Autodesk Inventor part; units mm, degrees
ref_plane "Work Plane2" through (8, 0, 0) normal (0, 0, 1) x (1, 0, 0)
ref_plane "Work Plane4" through (8, 0, 0) normal (0, 0, 1) x (1, 0, 0)
ref_plane "Work Plane5" through (11, -5, -9) normal (1, 0, 0) x (0, 1, 0)
ref_plane "Work Plane1" through (11, 2.9624, 8) normal (0, 0, -1) x (-1, 0, 0)
sketch "Sketch1" plane through (11, 2.9624, 8) normal (0, 0, -1) x (-1, 0, 0)
  arc A0 (0.0647, 1) -> (3.5, -0.2722) centre (5.5324, 10.4896) ccw
  line L0 (0, -2.9624) -> (0, 1)
  line L1 (3.5, -0.2722) -> (3.5, -2.9624)
  line L2 (0, -2.9624) -> (3.5, -2.9624)
  arc A1 (0, 1.0376) -> (11, 1) centre (5.5324, 10.4896) ccw
  line L3 (0, -7.9624) -> (0, 1.0376)
  line L4 (3.5, -0.2722) -> (3.5, -2.9624)
  line L5 (0, -2.9624) -> (3.5, -2.9624)
  line L6 (0, -2.9624) -> (0, 1.0376)
  arc A2 (0, 1.0376) -> (11, 1) centre (5.5324, 10.4896) ccw
  point P0 (11, -2.9624)
ref_plane "Work Plane2" through (8, 0, 0) normal (0, 0, 1) x (1, 0, 0)
ref_plane "Work Plane4" through (8, 0, 0) normal (0, 0, 1) x (1, 0, 0)
extrude "Extrusion1" add sketch "Sketch1" along normal up to surface (8 mm away)
ref_plane "Work Plane3" through (8, -5, 14.5) normal (-1, 0, 0) x (0, 0, 1)
ref_plane "Work Plane5" through (11, -5, -9) normal (1, 0, 0) x (0, 1, 0)
sketch "Sketch2" plane through (8, -5, 14.5) normal (-1, 0, 0) x (0, 0, 1)
  line L0 (-6.5, 5) -> (-14.5, 5)
  line L1 (-12, 5) -> (-12, 0)
  line L2 (-12, 5) -> (-12, 0)
  line L3 (-12, 5) -> (-9.4556, 5)
  line L4 (-12, 0) -> (-22.5, 0)
  line L5 (-22.5, 0) -> (-22.5, -26)
  line L6 (1.0444, 0) -> (1.0444, -26)
  line L7 (1.0444, -26) -> (-22.5, -26)
  line L8 (-22.5, 0) -> (-19.5, 0)
  line L9 (-19.5, 0) -> (-19.5, -3)
  line L10 (1.0444, -26) -> (1.0444, -23)
  line L11 (1.0444, -23) -> (-1.9556, -23)
  line L12 (-19.5, -3) -> (-1.9556, -3)
  line L13 (-1.9556, -3) -> (-1.9556, -23)
  line L14 (-1.9556, -23) -> (-19.5, -23)
  line L15 (-19.5, -23) -> (-19.5, -3)
  line L16 (1.0444, -26) -> (-0.9556, -26)
  line L17 (-0.9556, -26) -> (-2.9556, -26)
  line L18 (-22.5, 0) -> (-22.5, -4)
  line L19 (-22.5, -4) -> (-22.5, -2)
  line L20 (-22.5, -2) -> (-24.5, -2)
  line L21 (1.0444, 0) -> (1.0444, -4)
  line L22 (1.0444, -2) -> (3.0444, -2)
  arc A0 (-22.5, 0) -> (-22.5, -4) centre (-22.5, -2) ccw
  arc A1 (1.0444, -4) -> (1.0444, 0) centre (1.0444, -2) ccw
  line L23 (-9, 0) -> (-9, 5)
  line L24 (-12, 5) -> (-9, 5)
  line L25 (-9, 5) -> (-9, 0)
  line L26 (1.0444, 0) -> (-9, 0)
  line L27 (-22.5, -26) -> (-22.5, -24)
  line L28 (-22.5, -24) -> (-24.5, -24)
  line L29 (1.0444, -26) -> (1.0444, -24)
  line L30 (1.0444, -24) -> (3.0444, -24)
  line L31 (-22.5, -24) -> (-22.5, -22)
  line L32 (1.0444, -24) -> (1.0444, -22)
  arc A2 (-22.5, -22) -> (-22.5, -26) centre (-22.5, -24) ccw
  arc A3 (1.0444, -26) -> (1.0444, -22) centre (1.0444, -24) ccw
  line L33 (-19.5, -23) -> (-1.9556, -23)
  line L34 (-1.9556, -3) -> (-1.9556, -23)
  point P0 (-18.5, -26)
  dimension "d3" = 10.5
  dimension "d4" = 26
  dimension "d5" = 3
  dimension "d6" = 3
  dimension "d8" = 3
  dimension "d16" = 4
  dimension "d17" = 2
  dimension "d18" = 4
  dimension "d19" = 2
  dimension "d28" = 2
  dimension "d29" = 2
  dimension "d30" = 2
  dimension "d31" = 2
  dimension "d32" = 2
extrude "Extrusion2" add sketch "Sketch2" along normal up to surface (3.5 mm away) from surface at -3 contours L23 L26 L6 L11 L13 L12 L9 L4 L1 L0 | A1 L22 L6 | L22 A1 L6 | L9 L15 L14 L11 L6 L7 L5 L4 | L5 L20 A0 | A3 L30 L6 | L5 A0 L20 | A3 L6 L30 | L5 L28 A2 | L5 A2 L28
sketch "Sketch3" plane through (11, 0, 8) normal (1, 0, 0) x (0, 0, -1)
  arc A0 (-7.5444, -5) -> (-7.5444, -9) centre (-7.5444, -7) ccw
  arc A1 (16, -9) -> (16, -5) centre (16, -7) ccw
  circle A2 centre (16, -7) radius 1
  circle A3 centre (-7.5444, -7) radius 1
  arc A4 (-7.5444, -27) -> (-7.5444, -31) centre (-7.5444, -29) ccw
  arc A5 (16, -31) -> (16, -27) centre (16, -29) ccw
  circle A6 centre (16, -29) radius 1
  circle A7 centre (-7.5444, -29) radius 1
  point P0 (-5.5444, -31)
  dimension "d23" = 2
  dimension "d25" = 2
  dimension "d33" = 2
  dimension "d34" = 2
extrude "Extrusion3" cut sketch "Sketch3" against normal up to surface (3.5 mm away)
properties part number "back_pack_side_clip_in"
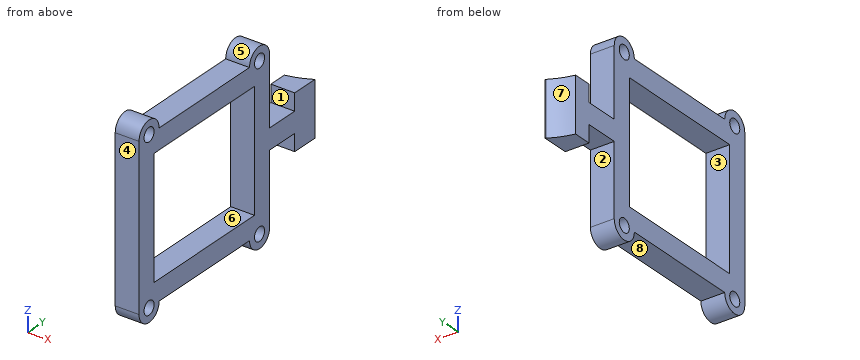
Input: part model. Units: mm. Frame: model coordinates. Face numbers are marked on the shaded views. A direction names the side the tool comes from. Give positions to 0.01 mm unless a question says otherwise; leave off trailing zeros. Write each loop counter-clockwise with the first axis right and the second up, starting at its lowest first coordinate (ties: lowest second). Pieces come first, ordered by that corner, then holes. Notation, with made-up numbers: (74.5, 11.5) - (103.5, 11.5) arc R21 cw to (103.5, 37.5) - close; hole circle Ø5 at (-20, 33). An arc over 180 degrees is marked (long way). Write item = value, one per line. Start each with the question number.
1. Section query A-A, the plane y = -29. Output: boundary loops of the cut face in (x, z), then the cut area to 3 significant figures.
2. Section query C-C, the plane x = 9.6. Output: boundary loops of the cut face in (y, z).
3. Section query B-B, the plane y = -23.5. Output: boundary loops of the cut face in (x, z), then the cut area to 3 significant figures.
4. First-contact query: pin 1 Ø1.8 at (x, z) = (10, 3.5) entering from +Y; pin 2 Ø1 at (x, z) = (10, -3.5) entering from +Y; pin 3 Ø2 at (x, y) = (10.5, -16) entering from +Z. Flat tips, straight axial feed; report the tip coordinate or a pass-through.
5. Section query D-D, the plane z = -5.5. Output: boundary loops of the cut face in (x, y), then the cut area to 3 significant figures.
6. Mould query, pull axis Z, two halves, no side actions, for the marked faces 5, 6, 7 and 8. Classes: released by +Z, released by -Z, zero draft, split by the parting line, or undercut.
7. Ray query, L1, parallel to Z at x = 7.95, y = -18.5; L2, parallel to Y at x = 8.45, z = 0.25; L3, parallel to Y at x = 10.75, z = 14.75. Return the intervals inside material, ascending.
8. Access query for the marked faces 1, 2, 3 and 4. Directions: +Z, -Z, +X, -X, +Y, -Y. A direction counts if a zero-diameter tool reaches every point of the face in a straight line with its end or side. Return the directions, or none.
Check sheet entries:
q1.outline = (7.5, -10) - (11, -10) - (11, -9) - (7.5, -9) - close; (7.5, -7) - (11, -7) - (11, 14.54) - (7.5, 14.54) - close; (7.5, 16.54) - (11, 16.54) - (11, 17.54) - (7.5, 17.54) - close
q1.area = 82.4 mm2
q2.outline = (-31, -8) arc R2 ccw to (-27, -8) - (-9, -8) arc R2 ccw to (-5, -8) - (-5, 2.5) - (0, 2.5) - (0, 0) - (3.31, 0) - (3.31, 8) - (0, 8) - (0, 5.5) - (-5, 5.5) - (-5, 15.54) arc R2 ccw to (-9, 15.54) - (-27, 15.54) arc R2 ccw to (-31, 15.54) - close; hole circle Ø2 at (-29, -8); hole circle Ø2 at (-29, 15.54); hole (-28, -5) - (-8, -5) - (-8, 12.54) - (-28, 12.54) - close; hole circle Ø2 at (-7, -8); hole circle Ø2 at (-7, 15.54)
q3.outline = (7.5, -8) - (11, -8) - (11, -5) - (7.5, -5) - close; (7.5, 12.54) - (11, 12.54) - (11, 15.54) - (7.5, 15.54) - close
q3.area = 21.0 mm2
q4.pin_1 = 3.94
q4.pin_2 = -5
q4.pin_3 = 15.54
q5.outline = (7.5, -31) - (11, -31) - (11, -5) - (7.5, -5) - close
q5.area = 91.0 mm2
q6.face_5 = released by +Z
q6.face_6 = undercut
q6.face_7 = zero draft
q6.face_8 = released by -Z
q7.L1 = -8 to -5, 12.54 to 15.54
q7.L2 = -31 to -28, -8 to -5, 0 to 2.91
q7.L3 = -31 to -29.61, -28.39 to -7.61, -6.39 to -5
q8.face_1 = +Z, +X, -X
q8.face_2 = -Z, +X, -X
q8.face_3 = +X, -X
q8.face_4 = +Z, -Z, +X, -X, -Y
